Here's how the part is built. I have some questions about the finished solid (model axes, mm). A direction names the side the tool comes from. Give positions to 0.01 mm unless a question says otherwise; leave off trailing zeros. Write each loop counter-clockwise with the first axis right and the second up, starting at its lowest first coordinate (ties: lowest second). Pieces come first, ordered by that corner, then holes. Notation, with made-up numbers: (3, -16.75) -> (47, -16.75) arc R25 cw to (47, -0.75) -> close; hole circle Ø9 at (-16, 18.25). An arc over 180 degrees is marked (long way). Answer as CSV lines item,"result". Start each with the question number.
from build123d import *

# Parameters (mm, degrees)
F0_W         = 18
F0_H         = 24
F1_DEPTH     = 34
F2_W         = 25
F2_H         = 13
F2_R         = 1.25
F3_DEPTH     = 16
F4_W         = 7
F4_H         = 20
F5_DEPTH     = 3
F6_R         = 1.25
F7_DEPTH     = 4
F8_T1_DEPTH  = 28
F8_T3_DEPTH  = 18
F8_T5_DEPTH  = 12
F8_S9_W      = 3
F8_S9_H      = 3
F8_T10_DEPTH = 3
F8_S15_W     = 3
F8_S15_H     = 3
F8_T16_DEPTH = 3
F8_S21_W     = 3
F8_S21_H     = 3
F8_T22_DEPTH = 3
F8_S27_W     = 3
F8_S27_H     = 3
F8_T28_DEPTH = 3
F8_S33_W     = 3
F8_S33_H     = 3
F8_T34_DEPTH = 3
F8_S39_W     = 3
F8_S39_H     = 3
F8_T40_DEPTH = 3
F8_S45_W     = 3
F8_S45_H     = 3
F8_T46_DEPTH = 3
F8_S51_W     = 3
F8_S51_H     = 3
F8_T52_DEPTH = 3
F9_R         = 3.5
F10_DEPTH    = 19
F11_R        = 1.25
F12_DEPTH    = 18.0010001


# Not quite as in the source:
# - a fillet or chamfer that OpenCascade refuses, or shapes differently, is made with other operations: its cross-section is extruded or revolved along the edge and cut away or added


with BuildPart() as f1:
    # F0 (on Front) → F1 (new body)
    with BuildSketch(Plane.XZ):
        with Locations((-10.5989521787, -5.2339873202)):
            Rectangle(F0_W, F0_H)
    extrude(amount=F1_DEPTH)

    # F2 (on face) → F3 (cut)
    with BuildSketch(Plane(origin=(-19.5989521787, 0, 0), x_dir=(0, -1, 0), z_dir=(-1, 0, 0))):
        with Locations((17, -7.2339873202)):
            Rectangle(F2_W, F2_H)
        with Locations((2.25, -7.2339873202)):
            Circle(F2_R)
        with Locations((31.75, -7.2339873202)):
            Circle(F2_R)
    extrude(amount=-F3_DEPTH, mode=Mode.SUBTRACT)

    # F4 (on face) → F5 (cut)
    with BuildSketch(Plane.XY.offset(6.7660126798)):
        with Locations((-10.5989521787, -17)):
            Rectangle(F4_W, F4_H)
    extrude(amount=-F5_DEPTH, mode=Mode.SUBTRACT)

    # F6 (on face) → F7 (cut)
    with BuildSketch(Plane.XY.offset(3.7660126798)):
        with Locations((-10.5989521787, -10.25)):
            Circle(F6_R)
        with Locations((-10.5989521787, -23.75)):
            Circle(F6_R)
    extrude(amount=-F7_DEPTH, mode=Mode.SUBTRACT)

    # F8: fillet of radius 3 on 12 edges, made by hand

    # F8_s2 → F8_t1 (cut)
    with BuildSketch(Plane.XZ.offset(3)):
        with BuildLine():
            ThreePointArc((-19.5989521787, 3.7660126798), (-18.7202725222, 5.8873330233), (-16.5989521787, 6.7660126798))
            Line((-16.5989521787, 6.7660126798), (-19.5989521787, 6.7660126798))
            Line((-19.5989521787, 6.7660126798), (-19.5989521787, 3.7660126798))
        make_face()
        with BuildLine():
            ThreePointArc((-16.5989521787, -17.2339873202), (-18.7202725222, -16.3553076638), (-19.5989521787, -14.2339873202))
            Line((-19.5989521787, -14.2339873202), (-19.5989521787, -17.2339873202))
            Line((-19.5989521787, -17.2339873202), (-16.5989521787, -17.2339873202))
        make_face()
        with BuildLine():
            ThreePointArc((-4.5989521787, -17.2339873202), (-2.4776318351, -16.3553076638), (-1.5989521787, -14.2339873202))
            Line((-1.5989521787, -14.2339873202), (-1.5989521787, -17.2339873202))
            Line((-1.5989521787, -17.2339873202), (-4.5989521787, -17.2339873202))
        make_face()
        with BuildLine():
            ThreePointArc((-1.5989521787, 3.7660126798), (-2.4776318351, 5.8873330233), (-4.5989521787, 6.7660126798))
            Line((-4.5989521787, 6.7660126798), (-1.5989521787, 6.7660126798))
            Line((-1.5989521787, 6.7660126798), (-1.5989521787, 3.7660126798))
        make_face()
    extrude(amount=F8_T1_DEPTH, mode=Mode.SUBTRACT)

    # F8_s4 → F8_t3 (cut)
    with BuildSketch(Plane.XY.offset(-14.2339873202)):
        with BuildLine():
            ThreePointArc((-19.5989521787, -31), (-18.7202725222, -33.1213203436), (-16.5989521787, -34))
            Line((-16.5989521787, -34), (-19.5989521787, -34))
            Line((-19.5989521787, -34), (-19.5989521787, -31))
        make_face()
        with BuildLine():
            ThreePointArc((-1.5989521787, -31), (-2.4776318351, -33.1213203436), (-4.5989521787, -34))
            Line((-4.5989521787, -34), (-1.5989521787, -34))
            Line((-1.5989521787, -34), (-1.5989521787, -31))
        make_face()
        with BuildLine():
            ThreePointArc((-19.5989521787, -3), (-18.7202725222, -0.8786796564), (-16.5989521787, 0))
            Line((-16.5989521787, 0), (-19.5989521787, 0))
            Line((-19.5989521787, 0), (-19.5989521787, -3))
        make_face()
        with BuildLine():
            ThreePointArc((-1.5989521787, -3), (-2.4776318351, -0.8786796564), (-4.5989521787, 0))
            Line((-4.5989521787, 0), (-1.5989521787, 0))
            Line((-1.5989521787, 0), (-1.5989521787, -3))
        make_face()
    extrude(amount=F8_T3_DEPTH, mode=Mode.SUBTRACT)

    # F8_s6 → F8_t5 (cut)
    with BuildSketch(Plane.YZ.offset(-16.5989521787)):
        with BuildLine():
            ThreePointArc((-31, -17.2339873202), (-33.1213203436, -16.3553076638), (-34, -14.2339873202))
            Line((-34, -14.2339873202), (-34, -17.2339873202))
            Line((-34, -17.2339873202), (-31, -17.2339873202))
        make_face()
        with BuildLine():
            ThreePointArc((0, 3.7660126798), (-0.8786796564, 5.8873330233), (-3, 6.7660126798))
            Line((-3, 6.7660126798), (0, 6.7660126798))
            Line((0, 6.7660126798), (0, 3.7660126798))
        make_face()
        with BuildLine():
            ThreePointArc((-34, 3.7660126798), (-33.1213203436, 5.8873330233), (-31, 6.7660126798))
            Line((-31, 6.7660126798), (-34, 6.7660126798))
            Line((-34, 6.7660126798), (-34, 3.7660126798))
        make_face()
        with BuildLine():
            ThreePointArc((-3, -17.2339873202), (-0.8786796564, -16.3553076638), (0, -14.2339873202))
            Line((0, -14.2339873202), (0, -17.2339873202))
            Line((0, -17.2339873202), (-3, -17.2339873202))
        make_face()
    extrude(amount=F8_T5_DEPTH, mode=Mode.SUBTRACT)


with BuildPart() as f8_tool8:
    # F8_s9 → F8_t10 (new body)
    with BuildSketch(Plane.YZ.offset(-16.5989521787)):
        with Locations((-1.5, 5.2660126798)):
            Rectangle(F8_S9_W, F8_S9_H)
    extrude(amount=-F8_T10_DEPTH)

    # F8_s11 → F8_t12 (revolve, cut)
    with BuildSketch(Plane(origin=(-16.5989521787, -3, 3.7660126798), x_dir=(0, -0.7071067812, -0.7071067812), z_dir=(0, 0.7071067812, -0.7071067812))):
        with BuildLine():
            ThreePointArc((0, -3), (3, 0), (0, 3))
            Line((0, 3), (0, -3))
        make_face()
    revolve(axis=Axis((-16.5989521787, -3, 3.7660126798), (-1, 0, 0)), mode=Mode.SUBTRACT)


with BuildPart() as f1_1:
    add(f1.part)

    # F8_t7: cut F8_tool8
    add(f8_tool8.part, mode=Mode.SUBTRACT)


with BuildPart() as f8_tool14:
    # F8_s15 → F8_t16 (new body)
    with BuildSketch(Plane.YZ.offset(-16.5989521787)):
        with Locations((-32.5, 5.2660126798)):
            Rectangle(F8_S15_W, F8_S15_H)
    extrude(amount=-F8_T16_DEPTH)

    # F8_s17 → F8_t18 (revolve, cut)
    with BuildSketch(Plane(origin=(-16.5989521787, -31, 3.7660126798), x_dir=(0, 0.7071067812, -0.7071067812), z_dir=(0, 0.7071067812, 0.7071067812))):
        with BuildLine():
            ThreePointArc((0, -3), (3, 0), (0, 3))
            Line((0, 3), (0, -3))
        make_face()
    revolve(axis=Axis((-16.5989521787, -31, 3.7660126798), (-1, 0, 0)), mode=Mode.SUBTRACT)


with BuildPart() as f1_2:
    add(f1_1.part)

    # F8_t13: cut F8_tool14
    add(f8_tool14.part, mode=Mode.SUBTRACT)


with BuildPart() as f8_tool20:
    # F8_s21 → F8_t22 (new body)
    with BuildSketch(Plane.XY.offset(-14.2339873202)):
        with Locations((-18.0989521787, -32.5)):
            Rectangle(F8_S21_W, F8_S21_H)
    extrude(amount=-F8_T22_DEPTH)

    # F8_s23 → F8_t24 (revolve, cut)
    with BuildSketch(Plane(origin=(-16.5989521787, -31, -14.2339873202), x_dir=(0.7071067812, 0.7071067812, 0), z_dir=(-0.7071067812, 0.7071067812, 0))):
        with BuildLine():
            ThreePointArc((0, -3), (3, 0), (0, 3))
            Line((0, 3), (0, -3))
        make_face()
    revolve(axis=Axis((-16.5989521787, -31, -14.2339873202), (0, 0, -1)), mode=Mode.SUBTRACT)


with BuildPart() as f1_3:
    add(f1_2.part)

    # F8_t19: cut F8_tool20
    add(f8_tool20.part, mode=Mode.SUBTRACT)


with BuildPart() as f8_tool26:
    # F8_s27 → F8_t28 (new body)
    with BuildSketch(Plane.XY.offset(-14.2339873202)):
        with Locations((-3.0989521787, -32.5)):
            Rectangle(F8_S27_W, F8_S27_H)
    extrude(amount=-F8_T28_DEPTH)

    # F8_s29 → F8_t30 (revolve, cut)
    with BuildSketch(Plane(origin=(-4.5989521787, -31, -14.2339873202), x_dir=(-0.7071067812, 0.7071067812, 0), z_dir=(-0.7071067812, -0.7071067812, 0))):
        with BuildLine():
            ThreePointArc((0, -3), (3, 0), (0, 3))
            Line((0, 3), (0, -3))
        make_face()
    revolve(axis=Axis((-4.5989521787, -31, -14.2339873202), (0, 0, -1)), mode=Mode.SUBTRACT)


with BuildPart() as f1_4:
    add(f1_3.part)

    # F8_t25: cut F8_tool26
    add(f8_tool26.part, mode=Mode.SUBTRACT)


with BuildPart() as f8_tool32:
    # F8_s33 → F8_t34 (new body)
    with BuildSketch(Plane.YZ.offset(-4.5989521787)):
        with Locations((-32.5, 5.2660126798)):
            Rectangle(F8_S33_W, F8_S33_H)
    extrude(amount=F8_T34_DEPTH)

    # F8_s35 → F8_t36 (revolve, cut)
    with BuildSketch(Plane(origin=(-4.5989521787, -31, 3.7660126798), x_dir=(0, 0.7071067812, -0.7071067812), z_dir=(0, -0.7071067812, -0.7071067812))):
        with BuildLine():
            ThreePointArc((0, -3), (3, 0), (0, 3))
            Line((0, 3), (0, -3))
        make_face()
    revolve(axis=Axis((-4.5989521787, -31, 3.7660126798), (1, 0, 0)), mode=Mode.SUBTRACT)


with BuildPart() as f1_5:
    add(f1_4.part)

    # F8_t31: cut F8_tool32
    add(f8_tool32.part, mode=Mode.SUBTRACT)


with BuildPart() as f8_tool38:
    # F8_s39 → F8_t40 (new body)
    with BuildSketch(Plane.XY.offset(-14.2339873202)):
        with Locations((-18.0989521787, -1.5)):
            Rectangle(F8_S39_W, F8_S39_H)
    extrude(amount=-F8_T40_DEPTH)

    # F8_s41 → F8_t42 (revolve, cut)
    with BuildSketch(Plane(origin=(-16.5989521787, -3, -14.2339873202), x_dir=(0.7071067812, -0.7071067812, 0), z_dir=(0.7071067812, 0.7071067812, 0))):
        with BuildLine():
            ThreePointArc((0, -3), (3, 0), (0, 3))
            Line((0, 3), (0, -3))
        make_face()
    revolve(axis=Axis((-16.5989521787, -3, -14.2339873202), (0, 0, -1)), mode=Mode.SUBTRACT)


with BuildPart() as f1_6:
    add(f1_5.part)

    # F8_t37: cut F8_tool38
    add(f8_tool38.part, mode=Mode.SUBTRACT)


with BuildPart() as f8_tool44:
    # F8_s45 → F8_t46 (new body)
    with BuildSketch(Plane.XY.offset(-14.2339873202)):
        with Locations((-3.0989521787, -1.5)):
            Rectangle(F8_S45_W, F8_S45_H)
    extrude(amount=-F8_T46_DEPTH)

    # F8_s47 → F8_t48 (revolve, cut)
    with BuildSketch(Plane(origin=(-4.5989521787, -3, -14.2339873202), x_dir=(-0.7071067812, -0.7071067812, 0), z_dir=(0.7071067812, -0.7071067812, 0))):
        with BuildLine():
            ThreePointArc((0, -3), (3, 0), (0, 3))
            Line((0, 3), (0, -3))
        make_face()
    revolve(axis=Axis((-4.5989521787, -3, -14.2339873202), (0, 0, -1)), mode=Mode.SUBTRACT)


with BuildPart() as f1_7:
    add(f1_6.part)

    # F8_t43: cut F8_tool44
    add(f8_tool44.part, mode=Mode.SUBTRACT)


with BuildPart() as f8_tool50:
    # F8_s51 → F8_t52 (new body)
    with BuildSketch(Plane.YZ.offset(-4.5989521787)):
        with Locations((-1.5, 5.2660126798)):
            Rectangle(F8_S51_W, F8_S51_H)
    extrude(amount=F8_T52_DEPTH)

    # F8_s53 → F8_t54 (revolve, cut)
    with BuildSketch(Plane(origin=(-4.5989521787, -3, 3.7660126798), x_dir=(0, -0.7071067812, -0.7071067812), z_dir=(0, -0.7071067812, 0.7071067812))):
        with BuildLine():
            ThreePointArc((0, -3), (3, 0), (0, 3))
            Line((0, 3), (0, -3))
        make_face()
    revolve(axis=Axis((-4.5989521787, -3, 3.7660126798), (1, 0, 0)), mode=Mode.SUBTRACT)


with BuildPart() as f1_8:
    add(f1_7.part)

    # F8_t49: cut F8_tool50
    add(f8_tool50.part, mode=Mode.SUBTRACT)

    # F9 (on face) → F10 (cut)
    with BuildSketch(Plane(origin=(0, 0, -17.2339873202), x_dir=(1, 0, 0), z_dir=(0, 0, -1))):
        with Locations((-10.5989521787, 10.5)):
            Circle(F9_R)
        with Locations((-10.5989521787, 23.5)):
            Circle(F9_R)
    extrude(amount=-F10_DEPTH, mode=Mode.SUBTRACT)

    # F11 (on face) → F12 (cut, through all)
    with BuildSketch(Plane.YZ.offset(-1.5989521787)):
        with Locations((-24.75, -5.2339873202)):
            Circle(F11_R)
    extrude(amount=-F12_DEPTH, mode=Mode.SUBTRACT)


solid = f1_8.part
Item 1: We'd pull the mould along Y, two halves only. Please class faces 1 (the face through (-9, -11, 1.766)), 2 (the face through (-2.5, -16.8, -16.38)), 3 (the face through (-2.454, -0.902, -5.36)): released by +Y, released by -Y, zero draft, split by the parting line, or undercut.
Item 2: If we section it at A-A (z = 1): Please give me the cut outline in (x, y).
Item 3: If we section it at D-D (z = -9.75): Please give me the cut outline in (x, y), and give its area (3 significant figures).
Item 4: If I drill on line 1 (Y direction, x = -13, z = -7.25); line 2 (Z direction, x = -13, y = -15.5); line 3 (Z direction, x = -14.75, y = -25), over which ranges is the centre line in solid material (lowest first)? Write a range as [from, to].
Item 5: For faces 4 (the face through (-11.358, -7.083, -15.508)), 5 (the face through (-14.099, -17, 5)), 6 (the face through (-2.454, -33.098, -5.36)), 7 (the face through (-11.71, -32.33, -8.34)), which set-ups out of +Z, -Z, +X, -X, +Y, -Y let a thin tool reach every point of the face, with its end or its side?
Item 6: If we section it at B-B (x = -8.75): State how many separate pieces and enclosed holes the cut face has, and give its area (3 significant figures).
Item 7: I'm going to push flat-ended pins straight in: pin 1 (1.5 mm diameter, centred on y = -24.75, z = -5.23, fed in from -X); pin 2 (1.5 mm diameter, centred on y = -19, z = 5, fed in from -X); pin 3 (3.5 mm diameter, centred on y = -13.5, z = 6, fed in from +X); pin 4 (1.5 mm diameter, centred on x = -11.5, z = 5, fed in from +Y). Where does each tip first touch, or does it pass through?
Item 8: If we section it at C-C (y = -5): Please give me the cut outline in (x, z), and give its area (3 significant figures).
Final values:
1,face 1,"undercut"
1,face 2,"zero draft"
1,face 3,"released by +Y"
2,outline,"(-19.6, -31) arc R3 ccw to (-16.6, -34) -> (-4.6, -34) arc R3 ccw to (-1.6, -31) -> (-1.6, -3) arc R3 ccw to (-4.6, 0) -> (-16.6, 0) arc R3 ccw to (-19.6, -3) -> close; hole circle Ø7 at (-10.6, -23.5); hole circle Ø7 at (-10.6, -10.5)"
3,outline,"(-19.6, -31) arc R3 ccw to (-16.6, -34) -> (-4.6, -34) arc R3 ccw to (-1.6, -31) -> (-1.6, -3) arc R3 ccw to (-4.6, 0) -> (-16.6, 0) arc R3 ccw to (-19.6, -3) -> (-19.6, -4.5) -> (-3.6, -4.5) -> (-3.6, -29.5) -> (-19.6, -29.5) -> close"
3,area,"204 mm2"
4,line 1,"[-34, -33], [-30.5, -29.5], [-4.5, -3.5], [-1, 0]"
4,line 2,"[-17.23, -13.73], [-0.73, 3.77]"
4,line 3,"[-17.23, -13.73], [-0.73, 6.77]"
5,face 4,"-Z"
5,face 5,"+Z"
5,face 6,"+Z, -Z, +X, -Y"
5,face 7,"-X"
6,separate pieces,"2"
6,enclosed holes,"2"
6,area,"342 mm2"
7,pin 1,"through"
7,pin 2,"x = -19.56"
7,pin 3,"x = -1.64"
7,pin 4,"y = -0.04"
8,outline,"(-19.6, -14.23) arc R3 ccw to (-16.6, -17.23) -> (-4.6, -17.23) arc R3 ccw to (-1.6, -14.23) -> (-1.6, 3.77) arc R3 ccw to (-4.6, 6.77) -> (-16.6, 6.77) arc R3 ccw to (-19.6, 3.77) -> (-19.6, -0.73) -> (-3.6, -0.73) -> (-3.6, -13.73) -> (-19.6, -13.73) -> close"
8,area,"216 mm2"
